```python
from build123d import *

# Parameters (mm, degrees)
CYLINDER001_R     = 2.1
CYLINDER001_DEPTH = 10
CYLINDER_R        = 2.1
CYLINDER_DEPTH    = 10
EXTRUDE_DEPTH     = 10
CYLINDER002_R     = 1.8
CYLINDER002_DEPTH = 200
ARRAY_X_COUNT     = 2
ARRAY_X_PITCH     = 86
ARRAY_Z_COUNT     = 2
ARRAY_Z_PITCH     = 44
BOX001_W          = 102
BOX001_H          = 3
BOX001_DEPTH      = 60


with BuildPart() as hole_minus:
    # Cylinder001 → Cylinder001 (new body)
    with BuildSketch(Plane(origin=(18.1, 10, 10), x_dir=(1, 0, 0), z_dir=(0, -1, 0))):
        Circle(CYLINDER001_R)
    extrude(amount=CYLINDER001_DEPTH)


with BuildPart() as hole_plus:
    # Cylinder → Cylinder (new body)
    with BuildSketch(Plane(origin=(-18.1, 10, 10), x_dir=(1, 0, 0), z_dir=(0, -1, 0))):
        Circle(CYLINDER_R)
    extrude(amount=CYLINDER_DEPTH)


with BuildPart() as display_hole_extrude:
    # Sketch → Extrude (new body)
    with BuildSketch(Plane.XZ):
        Polygon((-36, 19.5), (36, 19.5), (36, 6.5), (38, 6.5), (38, -6.5), (36, -6.5), (36, -19.5), (-36, -19.5), (-36, -6.5), (-38, -6.5), (-38, 6.5), (-36, 6.5), align=None)
    extrude(amount=-EXTRUDE_DEPTH)


with BuildPart() as display_hole_extrude_1:
    # Extrude placement: moved
    add(display_hole_extrude.part.moved(Location((0, 0, 37))))


with BuildPart() as hole_fusion:
    # Cylinder002 → Cylinder002 (new body)
    with BuildSketch(Plane(origin=(-43, 200, 8), x_dir=(1, 0, 0), z_dir=(0, -1, 0))):
        Circle(CYLINDER002_R)
    extrude(amount=CYLINDER002_DEPTH)

    # Array X: hole fusion ×2


with BuildPart() as hole_fusion_1:
    add(hole_fusion.part)
    with Locations(*[(i * ARRAY_X_PITCH, 0, 0) for i in range(1, ARRAY_X_COUNT)]):
        add(hole_fusion.part)

    # Array Z: hole fusion ×2


with BuildPart() as hole_fusion_2:
    add(hole_fusion_1.part)
    with Locations(*[(0, 0, i * ARRAY_Z_PITCH) for i in range(1, ARRAY_Z_COUNT)]):
        add(hole_fusion_1.part)

    # Fusion: union hole_minus, hole_plus, display hole extrude
    add(hole_minus.part)
    add(hole_plus.part)
    add(display_hole_extrude_1.part)


with BuildPart() as front_panel_cut:
    # Box001 → Box001 (new body)
    with BuildSketch(Plane(origin=(-51, 0, 0), x_dir=(1, 0, 0), z_dir=(0, 0, 1))):
        with Locations((51, 1.5)):
            Rectangle(BOX001_W, BOX001_H)
    extrude(amount=BOX001_DEPTH)

    # Cut: cut hole fusion
    add(hole_fusion_2.part, mode=Mode.SUBTRACT)


solid = front_panel_cut.part
```
Part model, mm, in its own coordinate system. A direction names the side the tool comes from. Coordinates: 2 decimals unless noted, no trailing zeros. Write each loop counter-clockwise with the first axis right and the second up, starting at its lowest first coordinate (ties: lowest second). Pieces come first, ordered by that corner, then holes.
Item 1: Slice it at D-D (x = -18.1). Write the cut outline in (y, z), and give its area (3 significant figures).
Item 2: Mould opens along Z. For faces 1 (the face through (-1, 2, 60)), 2 (the face through (-1, 2, 0)), 3 (the face through (-37, 1, 43.5)), 4 (the face through (-1, 0, 16)) say: released by +Z, released by -Z, zero draft, split by the parting line, or undercut.
Item 3: Which spindle directions (+Z, -Z, +X, -X, +Y, -Y) get a long thin tool onto all of the face, cutting with end or side? Do faces 5 (the face through (37, 1, 30.5)), 6 (the face through (-1, 3, 16)). Say none if no direction does.
Item 4: Pin check, flat tip, straight feed: pin 1 (1.6 mm diameter, centred on x = -36.5, y = 1.5, fed in from -Z). Stop position of the tip, or through.
Item 5: Probe line 1 (X direction, y = 1.05, z = 10); line 2 (Z direction, x = -43, y = 1.85); line 3 (Z direction, x = 13.5, y = 0.6). List the from-to ranges inside material, lowest first.
Item 6: Slice it at B-B (z = 45). Write the cut outline in (x, y), and give its area (3 significant figures).
Item 7: Slice it at C-C (y = 0.65). Write the cut outline in (x, z).
Item 8: Slice it at A-A (x = 1). Write the cut outline in (y, z), and give its area (3 significant figures).
Results found:
1. outline: (0, 0) - (3, 0) - (3, 7.9) - (0, 7.9) - close; (0, 12.1) - (3, 12.1) - (3, 17.5) - (0, 17.5) - close; (0, 56.5) - (3, 56.5) - (3, 60) - (0, 60) - close
1. area: 50.4 mm2
2. face 1: released by +Z
2. face 2: released by -Z
2. face 3: undercut
2. face 4: zero draft
3. face 5: +Y, -Y
3. face 6: +Z, -Z, +X, -X, +Y
4. pin 1: stops at z = 0
5. line 1: x = -51 to -20.2, -16 to 16, 20.2 to 51
5. line 2: z = 0 to 6.2, 9.8 to 50.2, 53.8 to 60
5. line 3: z = 0 to 17.5, 56.5 to 60
6. outline: (-51, 0) - (-36, 0) - (-36, 3) - (-51, 3) - close; (36, 0) - (51, 0) - (51, 3) - (36, 3) - close
6. area: 90.0 mm2
7. outline: (-51, 0) - (51, 0) - (51, 60) - (-51, 60) - close; hole circle Ø3.6 at (-43, 8); hole circle Ø3.6 at (-43, 52); hole (-38, 30.5) - (-36, 30.5) - (-36, 17.5) - (36, 17.5) - (36, 30.5) - (38, 30.5) - (38, 43.5) - (36, 43.5) - (36, 56.5) - (-36, 56.5) - (-36, 43.5) - (-38, 43.5) - close; hole circle Ø4.2 at (-18.1, 10); hole circle Ø4.2 at (18.1, 10); hole circle Ø3.6 at (43, 8); hole circle Ø3.6 at (43, 52)
8. outline: (0, 0) - (3, 0) - (3, 17.5) - (0, 17.5) - close; (0, 56.5) - (3, 56.5) - (3, 60) - (0, 60) - close
8. area: 63.0 mm2
